from build123d import *

# Parameters (mm, degrees)
F0_W     = 914.4
F0_H     = 914.4
F1_DEPTH = 914.4
F2_W     = 914.4
F2_H     = 165.717466
F3_DEPTH = 76.2
F4_R     = 337.986579
F5_DEPTH = 30.48


with BuildPart() as f1:
    # F0 (on Top) → F1 (new body)
    with BuildSketch(Plane.XY):
        with Locations((4.173182, 88.613961)):
            Rectangle(F0_W, F0_H)
    extrude(amount=F1_DEPTH)

    # F2 (on face) → F3 (join)
    with BuildSketch(Plane.XY.offset(914.4)):
        with Locations((4.173182, 462.955228)):
            Rectangle(F2_W, F2_H)
    extrude(amount=F3_DEPTH)

    # F4 (on face) → F5 (join)
    with BuildSketch(Plane.XZ.offset(368.586039)):
        with Locations((0, 510.469079)):
            Circle(F4_R)
    extrude(amount=F5_DEPTH)


solid = f1.part
Source: CAD feature listing. Evaluate the final solid. Frame: model axes, mm. A direction names the side the tool comes from. Coordinates: 2 decimals unless noted, no trailing zeros. Order: outer loops, then holes, each group sorted by start corner. A loop starts at its lowest first (then second) coordinate and runs counter-clockwise, first axis right, second up. Notation, with made-up numbers: M 46,69 L 101,69 A23 ccw 101,86 Z; hole C 21,77 d1. An arc over 180 degrees is marked long. Write each question's results on one line, items separated by ' | '. Start each with the question number.
1. Section A-A, the plane x = 0. Return the cut outline in (y, z), then the cut area to 3 significant figures.
2. Reachability of faces 1 (the face through (461.373, 82, 488)), 2 (the face through (-2, 11, 914.4)), 3 (the face through (-249.11, -383.613, 738.896)) from +Z, -Z, +X, -X, +Y, -Y: full face, straight path, thin tool, end or side. Return the list, or none.
3. Material intervals for L1, parallel to Z at x = -282.5, y = 37.5; L2, parallel to Y at x = -315, z = 89.5, sorted ascending.
4. Section B-B, the plane z = 928. Return the cut outline in (x, y), then the cut area to 3 significant figures.
5. Section C-C, the plane x = -388. Return the cut outline in (y, z).
6. Pin query (flat end, axial travel): pin 1 (8 mm diameter, centred on x = 310.5, y = -64.5, fed in from -Z); pin 2 (23 mm diameter, centred on x = 210, z = 953.5, fed in from -Y); pin 3 (1 mm diameter, centred on x = 91.5, y = -76.5, fed in from +Z). Return the tip coordinate at first contact, or that it passes through.
7. Section D-D, the plane y = 66.5. Return the cut outline in (x, z).
Solution:
1) outline: M -399.07,172.48 L -368.59,172.48 L -368.59,0 L 545.81,0 L 545.81,990.6 L 380.1,990.6 L 380.1,914.4 L -368.59,914.4 L -368.59,848.46 L -399.07,848.46 Z | area: 869,000 mm²
2) face 1: +Z, -Z, +X, +Y, -Y | face 2: +Z, +X, -X, -Y | face 3: -Y
3) L1: 0 to 914.4 | L2: -368.59 to 545.81
4) outline: M -453.03,380.1 L 461.37,380.1 L 461.37,545.81 L -453.03,545.81 Z | area: 152,000 mm²
5) outline: M -368.59,0 L 545.81,0 L 545.81,990.6 L 380.1,990.6 L 380.1,914.4 L -368.59,914.4 Z
6) pin 1: z = 0 | pin 2: y = 380.1 | pin 3: z = 914.4
7) outline: M -453.03,0 L 461.37,0 L 461.37,914.4 L -453.03,914.4 Z
